Can you work these out from the drawing? Everything is in mm from the part's minimum corner. Coordinates: 2 decimals unless noted, no trailing zeros. Loops run counter-clockwise (first coordinate to the right, second up) from the corner with the lowest first, then second, coordinate; pieces in that order, holes last. Notation, with made-up numbers: M 2.5,-5 L 38.5,-5 A18 ccw 38.5,12 Z; hole C -30.5,54.5 d4. An arc over 180 degrees is marked long. Write each question's results on one line, items separated by ' | '.
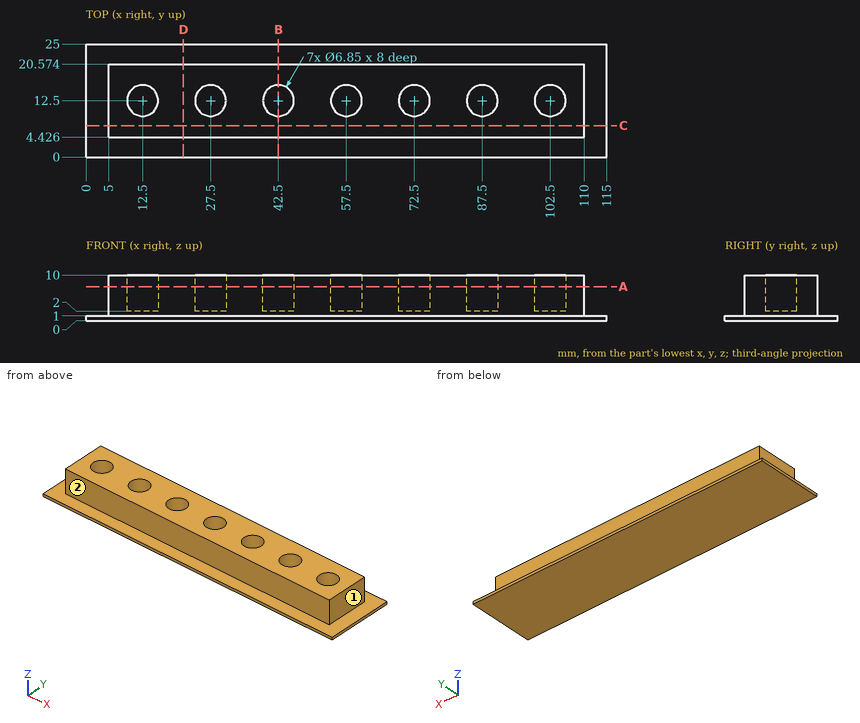
(1) If we mould it in two halves opening along Y, with no side actions, what happens to the marked faces 1 and 2? For each: released by +Y, released by -Y, zero draft, split by the parting line, or undercut.
Reported:
face 1: zero draft | face 2: released by -Y
(2) Will these pins go through, and if not, where does the flat tip stop? P1, Ø2, axis at y = 20, z = 8, coming from the +X side; P2, Ø1, axis at x = 15.5, y = 4, coming from the -Z side; P3, Ø6, axis at x = 102.5, y = 12.5, coming from the +Z side; P4, Ø1, axis at y = 4, z = 6.5, coming from the -X side.
Reported:
P1: stops at x = 110 | P2: stops at z = 0 | P3: stops at z = 2 | P4: stops at x = 5
(3) Imagine slicing it at C-C, the plane y = 7. List the corners of the cut face in (x, z) for me, and give its area (3 significant figures).
Reported:
outline: M 0,0 L 115,0 L 115,1 L 110,1 L 110,10 L 5,10 L 5,1 L 0,1 Z | area: 1,060 mm2
(4) Please list where these lines run through material, in increasing order: probe 1 along Y at (x, z) = (87.5, 3.5) (1 decimal); probe 2 along Z at (x, y) = (50.5, 3.5); probe 3 along Y at (x, z) = (18.5, 4.5) (1 decimal). Write a range as from..to.
Reported:
probe 1: y = 4.4..9.1, 15.9..20.6 | probe 2: z = 0..1 | probe 3: y = 4.4..20.6
(5) Imagine slicing it at B-B, the plane x = 42.5. List the corners of the cut face in (y, z) for me (1 decimal).
Reported:
outline: M 0,0 L 25,0 L 25,1 L 20.6,1 L 20.6,10 L 15.9,10 L 15.9,2 L 9.1,2 L 9.1,10 L 4.4,10 L 4.4,1 L 0,1 Z
(6) Imagine slicing it at A-A, the plane z = 7.5. State how many separate pieces and enclosed holes the cut face has, and give its area (3 significant figures).
Reported:
separate pieces: 1 | enclosed holes: 7 | area: 1,440 mm2
(7) Imagine slicing it at D-D, the plane x = 21.5. List the corners of the cut face in (y, z) for me (1 decimal).
Reported:
outline: M 0,0 L 25,0 L 25,1 L 20.6,1 L 20.6,10 L 4.4,10 L 4.4,1 L 0,1 Z
